Design review of the part built by this model. Coordinates are the model's own, in mm. A direction names the side the tool comes from. Give positions to 0.01 mm unless a question says otherwise; leave off trailing zeros. Order: outer loops, then holes, each group sorted by start corner. A loop starts at its lowest first (then second) coordinate and runs counter-clockwise, first axis right, second up. Notation, with made-up numbers: (-36, -21) -> (-3, -21) arc R18 ccw to (-3, -11) -> close; hole circle Ø9 at (-3, 46.5). An arc over 180 degrees is marked (long way). One line per item, written item: value.
from build123d import *

# Parameters (mm, degrees)
BOSS_EXTRUDE1_DEPTH = 1.5
FILLET1_R           = 5
SKETCH2_R           = 11.25
SKETCH2_R_2         = 1.5
CUT_EXTRUDE1_DEPTH  = 3
FILLET2_R           = 5
CUT_EXTRUDE2_REACH  = 160.212
SKETCH3_R           = 3


with BuildPart() as part:
    # Sketch1 → Boss-Extrude1 (new, symmetric)
    with BuildSketch(Plane(origin=(0, 0, 0), x_dir=(0, 1, 0), z_dir=(0, 0, 1))):
        Polygon((53.415, 0), (-53.415, 0), (-37, 149.099120638), (37, 149.099120638), align=None)
    extrude(amount=BOSS_EXTRUDE1_DEPTH, both=True)

    # Fillet1
    fillet1_edges = [part.edges().sort_by_distance(p)[0] for p in [
        (-149.099120638, -37, 0),
        (-149.099120638, 37, 0),
        (0, 53.415, 0),
        (0, -53.415, 0),
    ]]
    fillet(fillet1_edges, radius=FILLET1_R)

    # Sketch2 → Cut-Extrude1 (cut)
    with BuildSketch(Plane.XY.offset(1.5)):
        with Locations((-129.099120638, 0)):
            Circle(SKETCH2_R)
        Polygon((-56.099120638, 36.5), (-56.099120638, 0), (-56.099120638, -36.5), (-12.099120638, -36.5), (-12.099120638, 36.5), align=None)
        with BuildLine():
            Line((-102.849120638, 5), (-102.849120638, -5))
            Line((-102.849120638, -5), (-97.647079609, -5))
            ThreePointArc((-97.647079609, -5), (-76.849120638, 0), (-97.647079609, 5))
            Line((-97.647079609, 5), (-102.849120638, 5))
        make_face()
        with Locations((-7.099120638, 41.5)):
            Circle(SKETCH2_R_2)
        with Locations((-7.099120638, -41.5)):
            Circle(SKETCH2_R_2)
        with Locations((-61.099120638, -31.5)):
            Circle(SKETCH2_R_2)
        with Locations(Location((-61.099120638, 31.5, 0), (0, 0, 180))):
            Circle(SKETCH2_R_2)
    extrude(amount=-CUT_EXTRUDE1_DEPTH, mode=Mode.SUBTRACT)

    # Fillet2
    fillet2_edges = [part.edges().sort_by_distance(p)[0] for p in [
        (-56.099120638, -36.5, 0),
        (-56.099120638, 36.5, 0),
        (-12.099120638, 36.5, 0),
        (-12.099120638, -36.5, 0),
    ]]
    fillet(fillet2_edges, radius=FILLET2_R)

    # Sketch3 → Cut-Extrude2 (cut, up to next)
    with BuildSketch(Plane.XY.offset(1.5), mode=Mode.PRIVATE) as cut_extrude2_sk1:
        with Locations((-112.96609651, -23.875332325)):
            Circle(SKETCH3_R)
    cut_extrude2_tool1 = extrude(cut_extrude2_sk1.sketch, amount=-CUT_EXTRUDE2_REACH, mode=Mode.PRIVATE) & part.part
    # Sketch3 → Cut-Extrude2 (cut, up to next)
    with BuildSketch(Plane.XY.offset(1.5), mode=Mode.PRIVATE) as cut_extrude2_sk2:
        with Locations((-112.96609651, 23.875332325)):
            Circle(SKETCH3_R)
    cut_extrude2_tool2 = extrude(cut_extrude2_sk2.sketch, amount=-CUT_EXTRUDE2_REACH, mode=Mode.PRIVATE) & part.part
    add(cut_extrude2_tool1.solids().sort_by_distance((-112.966097, -23.875332, 1.5))[0], mode=Mode.SUBTRACT)
    add(cut_extrude2_tool2.solids().sort_by_distance((-112.966097, 23.875332, 1.5))[0], mode=Mode.SUBTRACT)


solid = part.part
Item 1: To check wall thickness, follow line 1 along X through (y, z) = (-15, -0.85); line 2 along X through (y, z) = (-30.5, 0.4); line 3 along X through (y, z) = (-2.5, -1.1). State the ranges of each line that lie inside material, in increasing order. Write a range as from..to.
Returned:
line 1: -149.1..-56.1, -12.1..0
line 2: -149.1..-62.22, -59.98..-56.1, -12.1..0
line 3: -149.1..-140.07, -118.13..-102.85, -77.14..-56.1, -12.1..0
Item 2: Add section C-C on z = -0.2. Count the separate pieces of the cut face and the enclosed holes in it, plus the area to 3 significant figures.
Returned:
separate pieces: 1
enclosed holes: 9
area: 9,360 mm²
Item 3: Clearance check with flat-ended pins moving along their axes: P1, Ø1.8, axis at x = -7.1, y = 41.5, coming from the -Z side; P2, Ø1.5, axis at x = -99.5, z = 0, coming from the -Y side. State where each tip first meets the part, or that it passes through.
Returned:
P1: through
P2: y = -42.54
Item 4: Draft analysis for pull direction X (two halves, no side actions). For faces 1 (the flat face through (-76, 1, 1.5)), 2 (the cylindrical face through (-60.293, -30.235, 0.021)), 3 (the flat face through (-149.099, 0, 0)), state which applies: pulls with the +X half, pulls with the -X half, needs draft (parallel to the pull), parting line crosses it, or undercut.
Returned:
face 1: needs draft
face 2: undercut
face 3: pulls with the -X half
Item 5: Add section A-A on x = -49. Give the boundary of the cut face in (y, z).
Returned:
outline: (-48.02, -1.5) -> (-36.5, -1.5) -> (-36.5, 1.5) -> (-48.02, 1.5) -> close; (36.5, -1.5) -> (48.02, -1.5) -> (48.02, 1.5) -> (36.5, 1.5) -> close
Item 6: Add section B-B on y = -41.5. Give the boundary of the cut face in (x, z), plus the area to 3 significant figures.
Returned:
outline: (-108.23, -1.5) -> (-8.6, -1.5) -> (-8.6, 1.5) -> (-108.23, 1.5) -> close; (-5.6, -1.5) -> (0, -1.5) -> (0, 1.5) -> (-5.6, 1.5) -> close
area: 316 mm²
Item 7: Machinability: for faces 4 (the flat face through (-76.07, 45.04, 0.02)), 5 (the cylindrical face through (-13.6, 35.07, -0.02)), which of the approach directions +Z, -Z, +X, -X, +Y, -Y give a long, thin tool a straight path to every point of the face, cutting with its end or side? Answer none if there is none.
Returned:
face 4: +Z, -Z, -X, +Y
face 5: +Z, -Z
